```python
from build123d import *

# Parameters (mm, degrees)
F0_R     = 75
F1_DEPTH = 80
F1_TAPER = -20
F2_R     = 95
F3_DEPTH = 70
F3_TAPER = 20
F4_R     = 30
F5_R     = 4.283
F6_R     = 72.5
F7_DEPTH = 5


# Not quite as in the source:
# - a fillet or chamfer that OpenCascade refuses, or shapes differently, is made with other operations: its cross-section is extruded or revolved along the edge and cut away or added


with BuildPart() as f1:
    # F0 (on Front) → F1 (new body)
    with BuildSketch(Plane.XZ):
        Circle(F0_R)
    extrude(amount=F1_DEPTH, taper=F1_TAPER)

    # F2 (on face) → F3 (cut)
    with BuildSketch(Plane.XZ.offset(80)):
        Circle(F2_R)
    extrude(amount=-F3_DEPTH, taper=F3_TAPER, mode=Mode.SUBTRACT)

    # F4
    f4_edges = [f1.edges().sort_by_distance(p)[0] for p in [
        (-69.522084, -10, 0),
    ]]
    fillet(f4_edges, radius=F4_R)

    # F5
    f5_edges = [f1.edges().sort_by_distance(p)[0] for p in [
        (-95, -80, 0),
        (-104.117619, -80, 0),
    ]]
    fillet(f5_edges, radius=F5_R)

    # F6 (on face) → F7 (cut)
    with BuildSketch(Plane(origin=(0, 0, 0), x_dir=(-1, 0, 0), z_dir=(0, 1, 0))):
        Circle(F6_R)
    extrude(amount=-F7_DEPTH, mode=Mode.SUBTRACT)

    # F8: fillet of radius 7 on 1 edges, made by hand

    # F8_s1 → F8_t2 (revolve)
    with BuildSketch(Plane.XY):
        with BuildLine():
            ThreePointArc((-72.5, 0), (-69.9750962002, -3.6124860802), (-65.7917960675, -5))
            Line((-65.7917960675, -5), (-72.5, -5))
            Line((-72.5, -5), (-72.5, 0))
        make_face()
    revolve(axis=Axis((0, -5, 0), (0, 1, 0)))


solid = f1.part
```
Check sheet for the modelled part. Datum: model origin and axes. Units: mm. Round coordinates to 2 decimals unless told otherwise and drop trailing zeros. Order: outer loops, then holes, each group sorted by start corner. A loop starts at its lowest first (then second) coordinate and runs counter-clockwise, first axis right, second up.
1) Section check C-C (y = -21). Record the boundary of the cut face in (x, z), and give its area (3 significant figures).
2) Scan lines: line 1 (Z direction, x = 14, y = -17.5); line 2 (Y direction, x = -33, z = -4.5); line 3 (X direction, y = -66.5, z = -3). Record each from-to range of solid material in increasing order.
3) Go/stop test with flat-tipped pins: pin 1 Ø1.5 at (x, z) = (19.5, -6) entering from +Y; pin 2 Ø10 at (y, z) = (-60.5, 52.5) entering from +X; pin 3 Ø8 at (x, y) = (38.5, -41) entering from +Z. Record where each tip stops, or that it passes through.
4) Mould release check, pull along X, two halves, no side actions. Record for faces 1 (the flat face through (-39.2, 0, 61.5)), 2 (the conical face through (-63.242, -12.895, -48.492)), 3 (the flat face through (1, -5, 1)): +X half, -X half, draft (parallel to the pull), parting line (faces both ways), or undercut.
5) Section check B-B (y = -46.5). Record the boundary of the cut face in (x, z).
Result:
1. outline: circle Ø165.29 at (0, 0); hole circle Ø143.46 at (0, 0)
1. area: 5,290 mm2
2. line 1: z = -80.16 to -66.91, 66.91 to 80.16
2. line 2: y = -10 to -5
2. line 3: x = -99.16 to -90.04, 90.04 to 99.16
3. pin 1: stops at y = -5
3. pin 2: stops at x = 85.29
3. pin 3: stops at z = 83.67
4. face 1: draft
4. face 2: parting line
4. face 3: undercut
5. outline: circle Ø183.85 at (0, 0); hole circle Ø165.61 at (0, 0)
